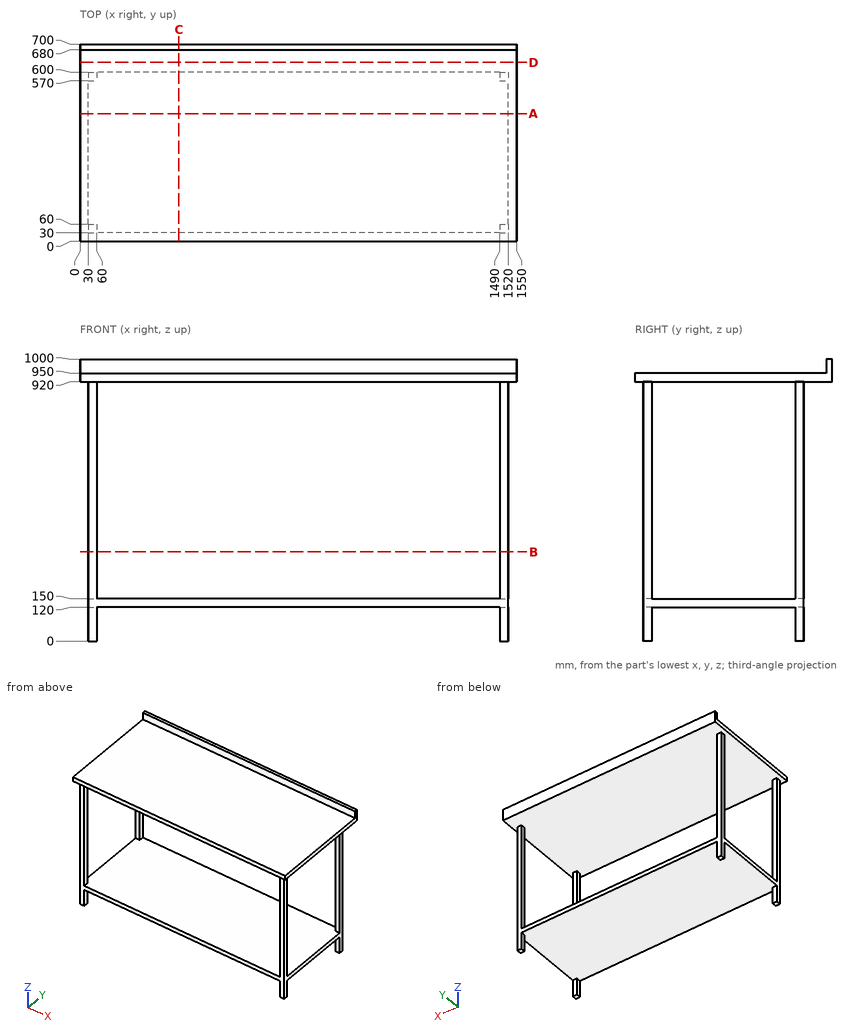
Could you check a few things on this drawing? It's one solid part, dimensions in mm from its lowest x, y, z. Round coordinates to 2 decimals unless told otherwise and drop trailing zeros. Order: outer loops, then holes, each group sorted by start corner. A loop starts at its lowest first (then second) coordinate and runs counter-clockwise, first axis right, second up. Notation, with made-up numbers: M -18,11 L 13,11 A25 cw 13,42 Z; hole C 48,26.25 d10. An arc over 180 degrees is marked long. Return JSON: item names as keys, results as strings. Group by question number.
1. If we section it at C-C on x = 351: List the corners of the cut face in (y, z) for me, then the cut area to 3 significant figures.
2. If we section it at A-A on y = 452.5: List the corners of the cut face in (x, z) for me.
3. If we section it at B-B on z = 316: List the corners of the cut face in (x, y) for me.
4. If we section it at D-D on y = 635: List the corners of the cut face in (x, z) for me, then the cut area to 3 significant figures.
5. Please list where these lines run through material, in increasing order: probe 1 along Z at (x, y) = (1075.5, 506); probe 2 along X at (y, z) = (47, 430); probe 3 along Y at (x, z) = (152.5, 126).
6. I'm going to push flat-ended pins straight in: pin 1 Ø15 at (y, z) = (588.5, 383.5) entering from -X; pin 2 Ø6 at (x, y) = (1177, 108) entering from +Z; pin 3 Ø9 at (x, z) = (1506, 351) entering from -Y. Where does each tip first touch, or does it pass through?
Reply:
{
 "1": {"outline": "M 0,920 L 700,920 L 700,1000 L 680,1000 L 680,950 L 0,950 Z; M 30,120 L 600,120 L 600,150 L 30,150 Z", "area": "39,100 mm^2"},
 "2": {"outline": "M 0,920 L 1550,920 L 1550,950 L 0,950 Z; M 30,120 L 1520,120 L 1520,150 L 30,150 Z"},
 "3": {"outline": "M 30,30 L 60,30 L 60,60 L 30,60 Z; M 30,570 L 60,570 L 60,600 L 30,600 Z; M 1490,30 L 1520,30 L 1520,60 L 1490,60 Z; M 1490,570 L 1520,570 L 1520,600 L 1490,600 Z"},
 "4": {"outline": "M 0,920 L 1550,920 L 1550,950 L 0,950 Z", "area": "46,500 mm^2"},
 "5": {"probe 1": "120 to 150, 920 to 950", "probe 2": "30 to 60, 1490 to 1520", "probe 3": "30 to 600"},
 "6": {"pin 1": "x = 30", "pin 2": "z = 950", "pin 3": "y = 30"}
}
